Source: CAD feature listing. Evaluate the final solid. Frame: model axes, mm. A direction names the side the tool comes from. Give positions to 0.01 mm unless a question says otherwise; leave off trailing zeros. Order: outer loops, then holes, each group sorted by start corner. A loop starts at its lowest first (then second) coordinate and runs counter-clockwise, first axis right, second up. Notation, with made-up numbers: (-26.5, -14.75) -> (15.5, -14.75) arc R28 cw to (15.5, 22.25) -> close; hole circle Ø5 at (67, -29.5). An arc over 180 degrees is marked (long way). Use CSV: the item, a comma, the result in double quotes.
```python
from build123d import *

# Parameters (mm, degrees)
CHAMFER1_SIZE      = 25.4
FILLET1_R          = 12.7
SKETCH3_W          = 30.48
SKETCH3_H          = 30.48
CUT_EXTRUDE1_DEPTH = 482.6
CIRPATTERN1_COUNT  = 36
FILLET2_R          = 12.7


with BuildPart() as part:
    # Sketch1 → Revolve1 (revolve)
    with BuildSketch(Plane.XY, mode=Mode.PRIVATE) as revolve1_sk:
        Polygon((254, 0), (508, 0), (508, 50.8), (419.1, 50.8), (419.1, 533.4), (508, 533.4), (508, 584.2), (254, 584.2), align=None)
    revolve(revolve1_sk.sketch.rotate(Axis((0, 0, 0), (0, 1, 0)), 90), axis=Axis((0, 0, 0), (0, 1, 0)))

    # Chamfer1
    chamfer1_edges = [part.edges().sort_by_distance(p)[0] for p in [
        (0, 584.2, 254),
    ]]
    chamfer(chamfer1_edges, length=CHAMFER1_SIZE)

    # Fillet1
    fillet1_edges = [part.edges().sort_by_distance(p)[0] for p in [
        (0, 584.2, 508),
        (0, 533.4, 508),
        (0, 50.8, 508),
        (0, 0, 508),
    ]]
    fillet(fillet1_edges, radius=FILLET1_R)

    # Sketch3 → Cut-Extrude1 (cut)
    with BuildSketch(Plane(origin=(0, 50.8, 0), x_dir=(1, 0, 0), z_dir=(0, 1, 0))):
        with Locations((30.48, 408.94)):
            Rectangle(SKETCH3_W, SKETCH3_H)
    cut_extrude1 = extrude(amount=CUT_EXTRUDE1_DEPTH, mode=Mode.SUBTRACT)

    # CirPattern1: Cut-Extrude1 ×36 about axis
    cirpattern1_axis = Axis((0, 0, 0), (0, 1, 0))
    for i in range(1, CIRPATTERN1_COUNT):
        add(cut_extrude1.rotate(cirpattern1_axis, i * 360 / CIRPATTERN1_COUNT), mode=Mode.SUBTRACT)

    # Fillet2
    fillet2_edges = [part.edges().sort_by_distance(p)[0] for p in [
        (0, 0, 254),
    ]]
    fillet(fillet2_edges, radius=FILLET2_R)


solid = part.part
```
1. Section query B-B on z = 0. Return loops of the section in (x, y).
Answer below:
outline,"(-508, 12.7) arc R12.7 ccw to (-495.3, 0) -> (-266.7, 0) arc R12.7 ccw to (-254, 12.7) -> (-254, 558.8) -> (-279.4, 584.2) -> (-495.3, 584.2) arc R12.7 ccw to (-508, 571.5) -> (-508, 546.1) arc R12.7 ccw to (-495.3, 533.4) -> (-419.1, 533.4) -> (-419.1, 50.8) -> (-495.3, 50.8) arc R12.7 ccw to (-508, 38.1) -> close; (254, 12.7) arc R12.7 ccw to (266.7, 0) -> (495.3, 0) arc R12.7 ccw to (508, 12.7) -> (508, 38.1) arc R12.7 ccw to (495.3, 50.8) -> (419.1, 50.8) -> (419.1, 533.4) -> (495.3, 533.4) arc R12.7 ccw to (508, 546.1) -> (508, 571.5) arc R12.7 ccw to (495.3, 584.2) -> (279.4, 584.2) -> (254, 558.8) -> close"
2. Access query for faces 1 (the cylindrical face through (-391.82, 295.48, 148.73)), 2 (the flat face through (55.508, 288.722, 402.563)), 3 (the cylindrical face through (-413.69, 295.48, -67.11)), 4 (the flat face through (-229.88, 288.722, -321.047)), 5 (the cylindrical face through (413.69, 295.48, 67.11)). Directions: +Z, -Z, +X, -X, +Y, -Y. A direction counts if a zero-diameter tool reaches every point of the face in a straight line with its end or side. Return the directions, or none.
Answer below:
face 1,"+Z, -X"
face 2,"+Z"
face 3,"-Z, -X"
face 4,"none"
face 5,"+Z, +X"
3. Mould query, pull axis Y, two halves, no side actions, for faces 6 (the conical face through (249.16, 560.03, 55.33)), 7 (the cylindrical face through (-324.714, 295.478, -264.964)). Classes: released by +Y, released by -Y, zero draft, split by the parting line, or undercut.
Answer below:
face 6,"released by +Y"
face 7,"undercut"
4. Pin query (flat end, axial travel): P1, Ø7.5, axis at x = 408, y = 244, coming from the +Z side; P2, Ø15, axis at y = 197.5, z = 33.5, coming from the +X side; P3, Ø15, axis at x = -23.5, y = 387, coming from the +Z side. Return the tip coordinate at first contact, or that it passes through.
Answer below:
P1,"stops at z = 87.74"
P2,"stops at x = 393.7"
P3,"stops at z = 393.7"
5. Section query A-A on x = 0. Return loops of the section in (y, z), plus the area to 3 significant figures.
Answer below:
outline,"(0, -495.3) arc R12.7 ccw to (12.7, -508) -> (38.1, -508) arc R12.7 ccw to (50.8, -495.3) -> (50.8, -419.1) -> (533.4, -419.1) -> (533.4, -495.3) arc R12.7 ccw to (546.1, -508) -> (571.5, -508) arc R12.7 ccw to (584.2, -495.3) -> (584.2, -279.4) -> (558.8, -254) -> (12.7, -254) arc R12.7 ccw to (0, -266.7) -> close; (0, 266.7) arc R12.7 ccw to (12.7, 254) -> (558.8, 254) -> (584.2, 279.4) -> (584.2, 495.3) arc R12.7 ccw to (571.5, 508) -> (546.1, 508) arc R12.7 ccw to (533.4, 495.3) -> (533.4, 419.1) -> (50.8, 419.1) -> (50.8, 495.3) arc R12.7 ccw to (38.1, 508) -> (12.7, 508) arc R12.7 ccw to (0, 495.3) -> close"
area,"210,000 mm²"
6. Ray query, line 1 along X through (y, z) = (321, 0); line 2 along X through (y, z) = (87.5, 221.5); line 3 along Y through (x, z) = (444, -151). Return the intervals inside material, ascending.
Answer below:
line 1,"x = -419.1 to -254, 254 to 419.1"
line 2,"x = -355.78 to -335.1, -328.08 to -124.31, 124.31 to 326.72, 353.17 to 355.78"
line 3,"y = 0 to 50.8, 533.4 to 584.2"
